```python
from build123d import *

# Parameters (mm, degrees)
SKETCH_W        = 100
SKETCH_H        = 160
PAD_DEPTH       = 24
SKETCH001_W     = 96
SKETCH001_H     = 156
POCKET_DEPTH    = 2
SKETCH002_W     = 92
SKETCH002_H     = 152
POCKET001_DEPTH = 22
SKETCH003_R     = 1
POCKET002_DEPTH = 24.001
SKETCH004_W     = 13
SKETCH004_H     = 13
SKETCH004_W_2   = 10
SKETCH004_H_2   = 4
SKETCH004_H_3   = 8
POCKET003_DEPTH = 10
SKETCH005_W     = 18
SKETCH005_H     = 1.5
POCKET004_DEPTH = 2
SKETCH007_R     = 9
POCKET005_DEPTH = 5
FILLET_R        = 1


with BuildPart() as part:
    # Sketch → Pad (new body)
    with BuildSketch(Plane.XY):
        Rectangle(SKETCH_W, SKETCH_H)
    extrude(amount=PAD_DEPTH)

    # Sketch001 → Pocket (cut)
    with BuildSketch(Plane.XY.offset(24)):
        Rectangle(SKETCH001_W, SKETCH001_H)
    extrude(amount=-POCKET_DEPTH, mode=Mode.SUBTRACT)

    # Sketch002 → Pocket001 (cut)
    with BuildSketch(Plane.XY.offset(24)):
        Rectangle(SKETCH002_W, SKETCH002_H)
    extrude(amount=-POCKET001_DEPTH, mode=Mode.SUBTRACT)

    # Sketch003 → Pocket002 (cut, through all)
    with BuildSketch(Plane.XY):
        with Locations((42, 72)):
            Circle(SKETCH003_R)
        with Locations((-42, 72)):
            Circle(SKETCH003_R)
        with Locations((42, -72)):
            Circle(SKETCH003_R)
        with Locations((-42, -72)):
            Circle(SKETCH003_R)
    extrude(amount=POCKET002_DEPTH, mode=Mode.SUBTRACT)

    # Sketch004 → Pocket003 (cut)
    with BuildSketch(Plane.XZ.offset(80)):
        with Locations((21.5, 13.5)):
            Rectangle(SKETCH004_W, SKETCH004_H)
        with Locations((-23, 18)):
            Rectangle(SKETCH004_W_2, SKETCH004_H_2)
        with Locations((-23, 9)):
            Rectangle(SKETCH004_W_2, SKETCH004_H_3)
    extrude(amount=-POCKET003_DEPTH, mode=Mode.SUBTRACT)

    # Sketch005 → Pocket004 (cut)
    with BuildSketch(Plane.XZ.offset(76)):
        with Locations((-23, 15.75)):
            Rectangle(SKETCH005_W, SKETCH005_H)
    extrude(amount=POCKET004_DEPTH, mode=Mode.SUBTRACT)

    # Sketch007 → Pocket005 (cut)
    with BuildSketch(Plane.XY):
        with Locations((34, 14)):
            Circle(SKETCH007_R)
        with Locations((-34, 14)):
            Circle(SKETCH007_R)
    extrude(amount=POCKET005_DEPTH, mode=Mode.SUBTRACT)

    # Fillet
    fillet_edges = [part.edges().sort_by_distance(p)[0] for p in [
        (-43, 14, 0),
    ]]
    fillet(fillet_edges, radius=FILLET_R)


solid = part.part
```
Part model, mm, in its own coordinate system. A direction names the side the tool comes from. Give positions to 0.01 mm unless a question says otherwise; leave off trailing zeros. Write each loop counter-clockwise with the first axis right and the second up, starting at its lowest first coordinate (ties: lowest second). Pieces come first, ordered by that corner, then holes. Notation, with made-up numbers: (1.5, 40) -> (47.5, 40) arc R22 ccw to (47.5, 52) -> close; hole circle Ø9 at (23.25, -0.5). An arc over 180 degrees is marked (long way). Put each result on its own line as item: value. Start each with the question number.
Item 1: Pin check, flat tip, straight feed: pin 1 Ø2 at (x, y) = (-8, 38.5) entering from +Z. Stop position of the tip, or through.
Item 2: Wall check: L1, parallel to X at y = 72, z = 1.4; L2, parallel to X at y = 14, z = 1.55; L3, parallel to Y at x = 42, z = 15.25. Give the ranges that are in metal, low to high. Write a range as [from, to].
Item 3: Cut at A-A (x = -34). List the corners of the cut face in (y, z), then the cut area to 3 significant figures.
Item 4: Cut at C-C (x = 4.5). List the corners of the cut face in (y, z).
Item 5: Cut at B-B (y = 14). List the corners of the cut face in (x, z), then the cut area to 3 significant figures.
Item 6: Cut at D-D (y = -44). List the corners of the cut face in (x, z).
Item 7: Pull direction Y, two halves, no side cores. Call faces 4 (the face through (-1, 1, 2)), 5 (the face through (-1, 80, 12)), 6 (the face through (28, -78, 13)): pulls with the +Y half, pulls with the -Y half, needs draft (parallel to the pull), parting line crosses it, or undercut.
Item 8: Which spindle directions (+Z, -Z, +X, -X, +Y, -Y) get a long thin tool onto all of the face, cutting with end or side? Do faces 1 (the face through (-48.4, 0.4, 24)), 2 (the face through (46, -1, 12)), 3 (the face through (21, -78, 20)). Say none if no direction does.
Answer list:
1. pin 1: stops at z = 2
2. L1: x = [-50, -43], [-41, 41], [43, 50]
2. L2: x = [-50, -43], [-25, 25], [43, 50]
2. L3: y = [-80, -76], [76, 80]
3. outline: (-80, 0) -> (4, 0) arc R1 ccw to (5, 1) -> (5, 2) -> (-76, 2) -> (-76, 22) -> (-78, 22) -> (-78, 24) -> (-80, 24) -> close; (23, 1) arc R1 ccw to (24, 0) -> (80, 0) -> (80, 24) -> (78, 24) -> (78, 22) -> (76, 22) -> (76, 2) -> (23, 2) -> close
3. area: 452 mm2
4. outline: (-80, 0) -> (80, 0) -> (80, 24) -> (78, 24) -> (78, 22) -> (76, 22) -> (76, 2) -> (-76, 2) -> (-76, 22) -> (-78, 22) -> (-78, 24) -> (-80, 24) -> close
5. outline: (-50, 0) -> (-44, 0) arc R1 ccw to (-43, 1) -> (-43, 2) -> (-46, 2) -> (-46, 22) -> (-48, 22) -> (-48, 24) -> (-50, 24) -> close; (-25, 1) arc R1 ccw to (-24, 0) -> (25, 0) -> (25, 2) -> (-25, 2) -> close; (43, 0) -> (50, 0) -> (50, 24) -> (48, 24) -> (48, 22) -> (46, 22) -> (46, 2) -> (43, 2) -> close
5. area: 296 mm2
6. outline: (-50, 0) -> (50, 0) -> (50, 24) -> (48, 24) -> (48, 22) -> (46, 22) -> (46, 2) -> (-46, 2) -> (-46, 22) -> (-48, 22) -> (-48, 24) -> (-50, 24) -> close
7. face 4: undercut
7. face 5: pulls with the +Y half
7. face 6: needs draft
8. face 1: +Z, +X, -X, +Y, -Y
8. face 2: +Z
8. face 3: -Y
